```python
from build123d import *

# Parameters (mm, degrees)
SKETCH1_R           = 6.39375
BOSS_EXTRUDE1_DEPTH = 4.2
BOSS_EXTRUDE2_DEPTH = 3
FILLET1_R           = 1
SKETCH3_R           = 1.5
CUT_EXTRUDE1_DEPTH  = 17.968242557
BOSS_EXTRUDE3_DEPTH = 3
CHAMFER1_SIZE       = 9
CHAMFER2_SIZE       = 6


with BuildPart() as part:
    # Sketch1 → Boss-Extrude1 (new body)
    with BuildSketch(Plane(origin=(0, 0, 0), x_dir=(1, 0, 0), z_dir=(0, 1, 0))):
        with Locations(Location((0, 0, 0), (0, 0, 270))):
            Circle(SKETCH1_R)
    extrude(amount=BOSS_EXTRUDE1_DEPTH)

    # Sketch2 → Boss-Extrude2 (add)
    with BuildSketch(Plane(origin=(0, 0, 0), x_dir=(1, 0, 0), z_dir=(0, 1, 0))):
        with BuildLine():
            Line((-1.433648629, 6.23094621), (-1.959549626, 8.516625387))
            add(Edge.make_bspline(
                [(-1.959549626, 8.516625387), (-1.745269759, 9.644412797), (-1.223586565, 10.731441367), (-0.488991141, 11.614711045)],
                knots=[0, 0, 0, 0, 1, 1, 1, 1], degree=3))
            ThreePointArc((-0.488991141, 11.614711045), (0, 11.625), (0.488991141, 11.614711045))
            add(Edge.make_bspline(
                [(1.959549626, 8.516625387), (1.745269759, 9.644412797), (1.223586565, 10.731441367), (0.488991141, 11.614711045)],
                knots=[0, 0, 0, 0, 1, 1, 1, 1], degree=3))
            Line((1.959549626, 8.516625387), (1.433648629, 6.23094621))
            ThreePointArc((1.433648629, 6.23094621), (0, 6.39375), (-1.433648629, 6.23094621))
        make_face()
        with BuildLine():
            Line((3.392201651, 5.419686986), (4.636552736, 7.407774392))
            add(Edge.make_bspline(
                [(4.636552736, 7.407774392), (5.585537608, 8.053721771), (6.723068605, 8.45348132), (7.86707199, 8.558609894)],
                knots=[0, 0, 0, 0, 1, 1, 1, 1], degree=3))
            ThreePointArc((7.86707199, 8.558609894), (8.220116331, 8.220116331), (8.558609894, 7.86707199))
            add(Edge.make_bspline(
                [(7.407774392, 4.636552736), (8.053721771, 5.585537608), (8.45348132, 6.723068605), (8.558609894, 7.86707199)],
                knots=[0, 0, 0, 0, 1, 1, 1, 1], degree=3))
            Line((7.407774392, 4.636552736), (5.419686986, 3.392201651))
            ThreePointArc((5.419686986, 3.392201651), (4.521063982, 4.521063982), (3.392201651, 5.419686986))
        make_face()
        with BuildLine():
            Line((6.23094621, 1.433648629), (8.516625387, 1.959549626))
            add(Edge.make_bspline(
                [(8.516625387, 1.959549626), (9.644412797, 1.745269759), (10.731441367, 1.223586565), (11.614711045, 0.488991141)],
                knots=[0, 0, 0, 0, 1, 1, 1, 1], degree=3))
            ThreePointArc((11.614711045, 0.488991141), (11.625, 0), (11.614711045, -0.488991141))
            add(Edge.make_bspline(
                [(8.516625387, -1.959549626), (9.644412797, -1.745269759), (10.731441367, -1.223586565), (11.614711045, -0.488991141)],
                knots=[0, 0, 0, 0, 1, 1, 1, 1], degree=3))
            Line((8.516625387, -1.959549626), (6.23094621, -1.433648629))
            ThreePointArc((6.23094621, -1.433648629), (6.39375, 0), (6.23094621, 1.433648629))
        make_face()
        with BuildLine():
            Line((5.419686986, -3.392201651), (7.407774392, -4.636552736))
            add(Edge.make_bspline(
                [(7.407774392, -4.636552736), (8.053721771, -5.585537608), (8.45348132, -6.723068605), (8.558609894, -7.86707199)],
                knots=[0, 0, 0, 0, 1, 1, 1, 1], degree=3))
            ThreePointArc((8.558609894, -7.86707199), (8.220116331, -8.220116331), (7.86707199, -8.558609894))
            add(Edge.make_bspline(
                [(4.636552736, -7.407774392), (5.585537608, -8.053721771), (6.723068605, -8.45348132), (7.86707199, -8.558609894)],
                knots=[0, 0, 0, 0, 1, 1, 1, 1], degree=3))
            Line((4.636552736, -7.407774392), (3.392201651, -5.419686986))
            ThreePointArc((3.392201651, -5.419686986), (4.521063982, -4.521063982), (5.419686986, -3.392201651))
        make_face()
        with BuildLine():
            Line((1.433648629, -6.23094621), (1.959549626, -8.516625387))
            add(Edge.make_bspline(
                [(1.959549626, -8.516625387), (1.745269759, -9.644412797), (1.223586565, -10.731441367), (0.488991141, -11.614711045)],
                knots=[0, 0, 0, 0, 1, 1, 1, 1], degree=3))
            ThreePointArc((0.488991141, -11.614711045), (0, -11.625), (-0.488991141, -11.614711045))
            add(Edge.make_bspline(
                [(-1.959549626, -8.516625387), (-1.745269759, -9.644412797), (-1.223586565, -10.731441367), (-0.488991141, -11.614711045)],
                knots=[0, 0, 0, 0, 1, 1, 1, 1], degree=3))
            Line((-1.959549626, -8.516625387), (-1.433648629, -6.23094621))
            ThreePointArc((-1.433648629, -6.23094621), (0, -6.39375), (1.433648629, -6.23094621))
        make_face()
        with BuildLine():
            Line((-3.392201651, -5.419686986), (-4.636552736, -7.407774392))
            add(Edge.make_bspline(
                [(-4.636552736, -7.407774392), (-5.585537608, -8.053721771), (-6.723068605, -8.45348132), (-7.86707199, -8.558609894)],
                knots=[0, 0, 0, 0, 1, 1, 1, 1], degree=3))
            ThreePointArc((-7.86707199, -8.558609894), (-8.220116331, -8.220116331), (-8.558609894, -7.86707199))
            add(Edge.make_bspline(
                [(-7.407774392, -4.636552736), (-8.053721771, -5.585537608), (-8.45348132, -6.723068605), (-8.558609894, -7.86707199)],
                knots=[0, 0, 0, 0, 1, 1, 1, 1], degree=3))
            Line((-7.407774392, -4.636552736), (-5.419686986, -3.392201651))
            ThreePointArc((-5.419686986, -3.392201651), (-4.521063982, -4.521063982), (-3.392201651, -5.419686986))
        make_face()
        with BuildLine():
            Line((-6.23094621, -1.433648629), (-8.516625387, -1.959549626))
            add(Edge.make_bspline(
                [(-8.516625387, -1.959549626), (-9.644412797, -1.745269759), (-10.731441367, -1.223586565), (-11.614711045, -0.488991141)],
                knots=[0, 0, 0, 0, 1, 1, 1, 1], degree=3))
            ThreePointArc((-11.614711045, -0.488991141), (-11.625, 0), (-11.614711045, 0.488991141))
            add(Edge.make_bspline(
                [(-8.516625387, 1.959549626), (-9.644412797, 1.745269759), (-10.731441367, 1.223586565), (-11.614711045, 0.488991141)],
                knots=[0, 0, 0, 0, 1, 1, 1, 1], degree=3))
            Line((-8.516625387, 1.959549626), (-6.23094621, 1.433648629))
            ThreePointArc((-6.23094621, 1.433648629), (-6.39375, 0), (-6.23094621, -1.433648629))
        make_face()
        with BuildLine():
            Line((-5.419686986, 3.392201651), (-7.407774392, 4.636552736))
            add(Edge.make_bspline(
                [(-7.407774392, 4.636552736), (-8.053721771, 5.585537608), (-8.45348132, 6.723068605), (-8.558609894, 7.86707199)],
                knots=[0, 0, 0, 0, 1, 1, 1, 1], degree=3))
            ThreePointArc((-8.558609894, 7.86707199), (-8.220116331, 8.220116331), (-7.86707199, 8.558609894))
            add(Edge.make_bspline(
                [(-4.636552736, 7.407774392), (-5.585537608, 8.053721771), (-6.723068605, 8.45348132), (-7.86707199, 8.558609894)],
                knots=[0, 0, 0, 0, 1, 1, 1, 1], degree=3))
            Line((-4.636552736, 7.407774392), (-3.392201651, 5.419686986))
            ThreePointArc((-3.392201651, 5.419686986), (-4.521063982, 4.521063982), (-5.419686986, 3.392201651))
        make_face()
    extrude(amount=BOSS_EXTRUDE2_DEPTH)

    # Fillet1
    fillet1_edges = [part.edges().sort_by_distance(p)[0] for p in [
        (-5.419686986, 1.5, -3.392201651),
        (-3.392201651, 1.5, -5.419686986),
        (3.392201651, 1.5, -5.419686986),
        (5.419686986, 1.5, -3.392201651),
        (6.23094621, 1.5, -1.433648629),
        (6.23094621, 1.5, 1.433648629),
        (5.419686986, 1.5, 3.392201651),
        (3.392201651, 1.5, 5.419686986),
        (1.433648629, 1.5, 6.23094621),
        (-1.433648629, 1.5, 6.23094621),
        (-3.392201651, 1.5, 5.419686986),
        (-5.419686986, 1.5, 3.392201651),
        (-1.433648629, 1.5, -6.23094621),
        (1.433648629, 1.5, -6.23094621),
        (-6.23094621, 1.5, 1.433648629),
        (-6.23094621, 1.5, -1.433648629),
    ]]
    fillet(fillet1_edges, radius=FILLET1_R)

    # Sketch3 → Cut-Extrude1 (cut, through all)
    with BuildSketch(Plane(origin=(0, 4.2, 0), x_dir=(1, 0, 0), z_dir=(0, 1, 0))):
        with Locations(Location((0, 0, 0), (0, 0, 270))):
            Circle(SKETCH3_R)
    extrude(amount=-CUT_EXTRUDE1_DEPTH, mode=Mode.SUBTRACT)

    # Sketch4 → Boss-Extrude3 (add)
    with BuildSketch(Plane.XZ):
        Polygon((1.425680775, -4.920105114), (-4.487148233, -2.470931146), (-13.518477237, -24.274488114), (-19.154142386, -21.940119176), (-21.603316353, -27.852948184), (-10.054822196, -32.636491089), align=None)
    extrude(amount=-BOSS_EXTRUDE3_DEPTH)

    # Chamfer1
    chamfer1_edges = [part.edges().sort_by_distance(p)[0] for p in [
        (-10.054822196, 1.5, -32.636491089),
    ]]
    chamfer(chamfer1_edges, length=CHAMFER1_SIZE)

    # Chamfer2
    chamfer2_edges = [part.edges().sort_by_distance(p)[0] for p in [
        (-13.518477237, 1.5, -24.274488114),
    ]]
    chamfer(chamfer2_edges, length=CHAMFER2_SIZE)


solid = part.part
```
The model under review builds one solid part; all positions refer to its coordinate system, in mm. A direction names the side the tool comes from. Coordinates: 2 decimals unless noted, no trailing zeros. Order: outer loops, then holes, each group sorted by start corner. A loop starts at its lowest first (then second) coordinate and runs counter-clockwise, first axis right, second up. Notation, with made-up numbers: M 58.25,-37.75 L 116.25,-37.75 A14 ccw 116.25,-16.75 Z; hole C 55.25,-7.75 d6. An arc over 180 degrees is marked long. One line per question, with ' | ' between items.
(1) For probe 1 along X at (y, z) = (2.3, 0) (3 decimals); probe 2 along X at (y, z) = (2.4, 8); probe 3 along X at (y, z) = (3.05, 0), list the stretches that pass through material, from the lowest coordinate up. Write a range as from..to.
Geometry results:
probe 1: x = -11.625..-1.5, 1.5..11.625 | probe 2: x = -8.43..-5.71, -1.84..1.84, 5.71..8.43 | probe 3: x = -6.39..-1.5, 1.5..6.39
(2) Machinability: for faces 1 (the face through (6, 3, 6)), 2 (the face through (6.8, 1.479, 4.256)), 3 (the face through (-7.82, 1.48, 1.8)), 4 (the face through (4.27, 1.48, 6.82)), which of the approach directions +Z, -Z, +X, -X, +Y, -Y give a long, thin tool a straight path to every point of the face, cutting with its end or side? Answer none if there is none.
Geometry results:
face 1: +Z, +X, +Y | face 2: +X, +Y, -Y | face 3: +Y, -Y | face 4: +Z, +Y, -Y
(3) Add section B-B, the plane z = 0. Write out the cut boundary in (x, y) (3 decimals), then the cut area to 3 significant figures.
Geometry results:
outline: M -11.625,0 L -1.5,0 L -1.5,4.2 L -6.394,4.2 L -6.394,3 L -11.625,3 Z; M 1.5,0 L 11.625,0 L 11.625,3 L 6.394,3 L 6.394,4.2 L 1.5,4.2 Z | area: 72.5 mm²
(4) Add section A-A, the plane x = 0. Write out the cut boundary in (y, z) (3 decimals).
Geometry results:
outline: M 0,-11.625 L 3,-11.625 L 3,-6.394 L 4.2,-6.394 L 4.2,-1.5 L 0,-1.5 Z; M 0,1.5 L 4.2,1.5 L 4.2,6.394 L 3,6.394 L 3,11.625 L 0,11.625 Z
(5) Add section C-C, the plane x = -16.5. Write out the cut boundary in (y, z).
Geometry results:
outline: M 0,-28.42 L 3,-28.42 L 3,-20.92 L 0,-20.92 Z
(6) The part is to be moulded in two halves that separate along X. For faces 5 (the face through (9, 3, 0)), 6 (the face through (-5.78, 1.52, 3.32)), 7 (the face through (4.256, 1.479, -6.8)), say which applies: +X half, -X half, draft (parallel to the pull), parting line (faces both ways), or undercut.
Geometry results:
face 5: draft | face 6: -X half | face 7: undercut
(7) Insertion check: pin 1 (2.5 mm diameter, centred on x = -9, z = 0, fed in from +Y); pin 2 (2 mm diameter, centred on x = -4, y = 2, fed in from +Z); pin 3 (1 mm diameter, centred on y = 0.5, z = 5, fed in from +X). Each pin has a flat end and moves straight along its axis. Give the tip position at first contact, or say it passes through.
Geometry results:
pin 1: stops at y = 3 | pin 2: stops at z = 7.64 | pin 3: stops at x = 7.9
(8) Add section D-D, the plane z = -13. Write out the cut boundary in (x, y).
Geometry results:
outline: M -8.85,0 L -1.92,0 L -1.92,3 L -8.85,3 Z
